Geometry: final body of the model. Coordinates: model frame, mm. Give positions to 0.01 mm unless a question says otherwise; leave off trailing zeros. Order: outer loops, then holes, each group sorted by start corner. A loop starts at its lowest first (then second) coordinate and runs counter-clockwise, first axis right, second up. Notation, with made-up numbers: (31, -32) -> (52, -32) arc R19 ccw to (52, -19) -> close; hole circle Ø4 at (-6, 26). An arc over 180 degrees is marked (long way). Write item = value, one per line.
```python
from build123d import *

# Parameters (mm, degrees)
ESQUISSE1_W             = 25
ESQUISSE1_H             = 25
BOSS_EXTRU_1_DEPTH      = 5
ENL_V_MAT_EXTRU_1_REACH = 37.707
ESQUISSE2_R             = 4.3
CONG_2_R                = 1
CONG_3_R                = 1


with BuildPart() as part:
    # Esquisse1 → Boss.-Extru.1 (new body)
    with BuildSketch(Plane(origin=(0, 0, 0), x_dir=(1, 0, 0), z_dir=(0, 1, 0))):
        with Locations((-12.5, 12.5)):
            Rectangle(ESQUISSE1_W, ESQUISSE1_H)
    extrude(amount=BOSS_EXTRU_1_DEPTH)

    # Esquisse2 → Enlèv. mat.-Extru.1 (cut, up to next)
    with BuildSketch(Plane(origin=(0, 5, 0), x_dir=(1, 0, 0), z_dir=(0, 1, 0)), mode=Mode.PRIVATE) as enl_v_mat_extru_1_sk1:
        with Locations(Location((-12.5, 12.5, 0), (0, 0, 270))):
            Circle(ESQUISSE2_R)
    enl_v_mat_extru_1_tool1 = extrude(enl_v_mat_extru_1_sk1.sketch, amount=-ENL_V_MAT_EXTRU_1_REACH, mode=Mode.PRIVATE) & part.part
    add(enl_v_mat_extru_1_tool1.solids().sort_by_distance((-12.5, 5, -12.5))[0], mode=Mode.SUBTRACT)

    # Congé2
    cong_2_edges = [part.edges().sort_by_distance(p)[0] for p in [
        (-12.5, 0, -16.8),
    ]]
    fillet(cong_2_edges, radius=CONG_2_R)

    # Congé3
    cong_3_edges = [part.edges().sort_by_distance(p)[0] for p in [
        (-12.5, 5, -16.8),
    ]]
    fillet(cong_3_edges, radius=CONG_3_R)


solid = part.part
```
1) Section query B-B (x = -12.5). Output: boundary loops of the cut face in (y, z), plus the area to 3 significant figures.
Check sheet entries:
outline = (0, -25) -> (5, -25) -> (5, -17.8) arc R1 ccw to (4, -16.8) -> (1, -16.8) arc R1 ccw to (0, -17.8) -> close; (0, -7.2) arc R1 ccw to (1, -8.2) -> (4, -8.2) arc R1 ccw to (5, -7.2) -> (5, 0) -> (0, 0) -> close
area = 81.1 mm²
2) First-contact query: P1, Ø14, axis at x = -12.5, z = -12.5, coming from the -Y side. Flat tip, straight axial feed; report the tip coordinate or a pass-through.
Check sheet entries:
P1 = 0
3) Section query A-A (z = -12.5). Output: boundary loops of the cut face in (x, y).
Check sheet entries:
outline = (-25, 0) -> (-17.8, 0) arc R1 ccw to (-16.8, 1) -> (-16.8, 4) arc R1 ccw to (-17.8, 5) -> (-25, 5) -> close; (-8.2, 1) arc R1 ccw to (-7.2, 0) -> (0, 0) -> (0, 5) -> (-7.2, 5) arc R1 ccw to (-8.2, 4) -> close
4) Section query C-C (y = 2.05). Output: boundary loops of the cut face in (x, z).
Check sheet entries:
outline = (-25, -25) -> (0, -25) -> (0, 0) -> (-25, 0) -> close; hole circle Ø8.6 at (-12.5, -12.5)
5) Section query D-D (y = 0.3). Output: boundary loops of the cut face in (x, z), plus the area to 3 significant figures.
Check sheet entries:
outline = (-25, -25) -> (0, -25) -> (0, 0) -> (-25, 0) -> close; hole circle Ø9.17 at (-12.5, -12.5)
area = 559 mm²
6) Line query: line 1 (X direction, y = 2.7, z = -12.5); line 2 (Z direction, x = -11, y = 3.55); line 3 (X direction, y = 1.65, z = -13.25). Output: solid intervals per line, ascending. Write a range as from..to.
Check sheet entries:
line_1 = -25..-16.8, -8.2..0
line_2 = -25..-16.53, -8.47..0
line_3 = -25..-16.73, -8.27..0
7) Mould query, pull axis X, two halves, no side actions, for faces 1 (the face through (-25, 2, -12)), 2 (the face through (-7, 0, -13)), 3 (the face through (-12.311, 2.521, -16.796)), 4 (the face through (0, 2, -12)). Classes: +X half, -X half, draft (parallel to the pull), parting line (faces both ways), or undercut.
Check sheet entries:
face_1 = -X half
face_2 = draft
face_3 = undercut
face_4 = +X half
